Could you check a few things on this model? Use its own coordinates, in mm. Coordinates: 2 decimals unless noted, no trailing zeros. Write each loop counter-clockwise with the first axis right and the second up, starting at its lowest first coordinate (ties: lowest second). Pieces come first, ordered by that corner, then holes. Notation, with made-up numbers: (-12, -10) - (-5, -10) arc R11 cw to (-5, 11) - close; hole circle Ø5 at (5.5, 79). An arc over 180 degrees is marked (long way). Answer as a JSON object with one key per item and string values. Group by question number.
1) If we section it at B-B (z = -14.5): Write out the boundary of the cut face in (x, y), plus the area to 3 significant figures.
2) Please list where these lines run through material, in increasing order: line 1 along Z through (x, y) = (-11, -0.15); line 2 along Z through (x, y) = (62.25, 0.1); line 3 along X through (y, z) = (0.55, -30.5).
3) Will these pins go through, and if not, where does the flat tip stop? pin 1 Ø4.5 at (x, z) = (-11, -10) entering from +Y; pin 2 Ø2.5 at (x, z) = (-11, 10) entering from +Y; pin 3 Ø0.7 at (y, z) = (0, 15) entering from -X.
4) If we section it at C-C (z = -3): Write out the boundary of the cut face in (x, y), plus the area to 3 significant figures.
5) If we section it at A-A (y = -0.4): State how many separate pieces and enclosed holes the cut face has, plus the area to 3 significant figures.
```python
from build123d import *

# Parameters (mm, degrees)
PAD_DEPTH       = 0.7
PAD_DEPTH_BACK  = 0.7
SKETCH001_R     = 1.65
POCKET_DEPTH    = 1.401
SKETCH002_R     = 1.65
SKETCH002_W     = 10
SKETCH002_H     = 5
POCKET001_DEPTH = 1.401


with BuildPart() as part:
    # Sketch → Pad (new body, two sides)
    with BuildSketch(Plane.XZ) as pad_sk:
        with BuildLine():
            Line((-105, -41), (-105, -36))
            ThreePointArc((-105, -36), (-52.968759, -12.982946), (-35, 41))
            Line((-35, 41), (105, 41))
            Line((105, 41), (105, -41))
            Line((105, -41), (-105, -41))
        make_face()
    extrude(amount=PAD_DEPTH)
    extrude(pad_sk.sketch, amount=-PAD_DEPTH_BACK)

    # Sketch001 (on Face7 of Pad) → Pocket (cut, through all)
    with BuildSketch(Plane.XZ.offset(0.7)):
        with Locations((100, 30)):
            Circle(SKETCH001_R)
        with Locations((100, 10)):
            Circle(SKETCH001_R)
        with Locations((-11, 30)):
            Circle(SKETCH001_R)
        with Locations((-11, 10)):
            Circle(SKETCH001_R)
        with Locations((100, -30)):
            Circle(SKETCH001_R)
        with Locations((100, -10)):
            Circle(SKETCH001_R)
        with Locations((-11, -30)):
            Circle(SKETCH001_R)
        with Locations((-11, -10)):
            Circle(SKETCH001_R)
    extrude(amount=-POCKET_DEPTH, mode=Mode.SUBTRACT)

    # Sketch002 (on Face5 of Pocket) → Pocket001 (cut, through all)
    with BuildSketch(Plane.XZ.offset(0.7)):
        with Locations((42.75, 31)):
            Circle(SKETCH002_R)
        with Locations((62.25, 31)):
            Circle(SKETCH002_R)
        with Locations((52.5, 16)):
            Rectangle(SKETCH002_W, SKETCH002_H)
    extrude(amount=-POCKET001_DEPTH, mode=Mode.SUBTRACT)


solid = part.part
```
Here are the results:
{
 "1": {"outline": "(-54.39, -0.7) - (105, -0.7) - (105, 0.7) - (-54.39, 0.7) - close", "area": "223 mm²"},
 "2": {"line 1": "z = -41 to -31.65, -28.35 to -11.65, -8.35 to 8.35, 11.65 to 28.35, 31.65 to 41", "line 2": "z = -41 to 29.35, 32.65 to 41", "line 3": "x = -77.74 to -12.57, -9.43 to 98.43, 101.57 to 105"},
 "3": {"pin 1": "stops at y = 0.7", "pin 2": "passes through", "pin 3": "stops at x = -37.49"},
 "4": {"outline": "(-45.4, -0.7) - (105, -0.7) - (105, 0.7) - (-45.4, 0.7) - close", "area": "211 mm²"},
 "5": {"separate pieces": "1", "enclosed holes": "11", "area": "12,700 mm²"}
}
